Input: part model. Units: mm. Frame: model coordinates. Round coordinates to 2 decimals unless told otherwise and drop trailing zeros. Loops run counter-clockwise (first coordinate to the right, second up) from the corner with the lowest first, then second, coordinate; pieces in that order, holes last.
1) Section C-C, the plane z = 2.75. State how many separate pieces and enclosed holes the cut face has, and give its area (3 significant figures).
2) Ray query, line 1 along Y through (x, z) = (-0.5, 1); line 2 along Y through (x, z) = (12, 5.25); line 3 along Y through (x, z) = (16, 3.75). Return the intervals inside material, ascending.
3) First-contact query: pin 1 (2.5 mm diameter, centred on x = -26.99, y = -41.53, fed in from -Z); pin 2 (1.5 mm diameter, centred on x = 10.5, z = 1, fed in from -Y). Flat tips, straight axial feed; report the tip coordinate or a pass-through.
4) Section A-A, the plane y = 0. Return loops of the section in (x, z) (3 decimals), and give its area (3 significant figures).
5) Draft query along X for faces 1 (the face through (-12.146, 47.678, 3.757)), 2 (the face through (-7.109, 54.145, 3.757)), 3 (the face through (36, 1, 7.62)). Return one class per face: pulls with the +X half, pulls with the -X half, needs draft (parallel to the pull), parting line crosses it, or undercut.
from build123d import *

# Parameters (mm, degrees)
SKETCH1_R           = 54.61
SKETCH1_R_2         = 34.925
BOSS_EXTRUDE1_DEPTH = 7.62
SKETCH3_R           = 2.0193
CUT_EXTRUDE1_DEPTH  = 8.62


with BuildPart() as part:
    # Sketch1 → Boss-Extrude1 (new body)
    with BuildSketch(Plane.XY):
        Circle(SKETCH1_R)
        Circle(SKETCH1_R_2, mode=Mode.SUBTRACT)
    extrude(amount=BOSS_EXTRUDE1_DEPTH)

    # Sketch3 → Cut-Extrude1 (cut, through all)
    with BuildSketch(Plane(origin=(0, 0, 0), x_dir=(-1, 0, 0), z_dir=(0, 0, -1))):
        with Locations((41.529703671, 26.990824607)):
            Circle(SKETCH3_R)
        with Locations((10.280539977, 48.451330196)):
            Circle(SKETCH3_R)
        with Locations((-26.990824607, 41.529703671)):
            Circle(SKETCH3_R)
        with Locations((-48.451330196, 10.280539977)):
            Circle(SKETCH3_R)
        with Locations((-41.529703671, -26.990824607)):
            Circle(SKETCH3_R)
        with Locations((-10.280539977, -48.451330196)):
            Circle(SKETCH3_R)
        with Locations((26.990824607, -41.529703671)):
            Circle(SKETCH3_R)
        with Locations((48.451330196, -10.280539977)):
            Circle(SKETCH3_R)
    extrude(amount=-CUT_EXTRUDE1_DEPTH, mode=Mode.SUBTRACT)


solid = part.part
Final values:
1. separate pieces: 1
1. enclosed holes: 9
1. area: 5,430 mm2
2. line 1: y = -54.61 to -34.92, 34.92 to 54.61
2. line 2: y = -53.28 to -49.51, -47.39 to -32.8, 32.8 to 53.28
2. line 3: y = -52.21 to -31.04, 31.04 to 52.21
3. pin 1: passes through
3. pin 2: stops at y = -53.73
4. outline: (-54.61, 0) - (-34.925, 0) - (-34.925, 7.62) - (-54.61, 7.62) - close; (34.925, 0) - (54.61, 0) - (54.61, 7.62) - (34.925, 7.62) - close
4. area: 300 mm2
5. face 1: undercut
5. face 2: parting line crosses it
5. face 3: needs draft
